```python
from build123d import *

# Parameters (mm, degrees)
SKETCH_1_R          = 5
EXTRUDE_1_DEPTH     = 5
SKETCH_3_W          = 5
SKETCH_3_H          = 8
EXTRUDE_2_DEPTH     = 15
SKETCH_2_R          = 2
CUT_EXTRUDE_1_DEPTH = 30
SKETCH_6_W          = 5
SKETCH_6_H          = 8
EXTRUDE_4_DEPTH     = 25
SKETCH_7_W          = 5
SKETCH_7_H          = 8
EXTRUDE_5_DEPTH     = 21
SKETCH_8_W          = 15
SKETCH_8_H          = 15
EXTRUDE_6_DEPTH     = 5
FILLET_2_R          = 2
SKETCH_9_R          = 2.15
CUT_EXTRUDE_2_DEPTH = 10
FILLET_3_R          = 5


with BuildPart() as part:
    # 草图1 → 凸台-拉伸1 (new body)
    with BuildSketch(Plane.XY):
        Circle(SKETCH_1_R)
    extrude(amount=EXTRUDE_1_DEPTH)

    # 草图3 → 凸台-拉伸2 (add)
    with BuildSketch(Plane(origin=(0, 0, 0), x_dir=(0, 0, -1), z_dir=(1, 0, 0))):
        with Locations((-2.5, 0)):
            Rectangle(SKETCH_3_W, SKETCH_3_H)
    extrude(amount=EXTRUDE_2_DEPTH)

    # 草图2 → 切除-拉伸1 (cut)
    with BuildSketch(Plane.XY.offset(5)):
        Circle(SKETCH_2_R)
    extrude(amount=-CUT_EXTRUDE_1_DEPTH, mode=Mode.SUBTRACT)

    # 草图6 → 凸台-拉伸4 (add)
    with BuildSketch(Plane.XY.offset(5)):
        with Locations((12.5, 0)):
            Rectangle(SKETCH_6_W, SKETCH_6_H)
    extrude(amount=EXTRUDE_4_DEPTH)

    # 草图7 → 凸台-拉伸5 (add)
    with BuildSketch(Plane(origin=(15, 0, 0), x_dir=(0, 0, -1), z_dir=(1, 0, 0))):
        with Locations((-27.5, 0)):
            Rectangle(SKETCH_7_W, SKETCH_7_H)
    extrude(amount=EXTRUDE_5_DEPTH)

    # 镜向2: part across plane


with BuildPart() as part_1:
    add(part.part)
    add(part.part.mirror(Plane(origin=(36, 0, 0), x_dir=(0, 0, 1), z_dir=(1, 0, 0))))

    # 草图8 → 凸台-拉伸6 (add)
    with BuildSketch(Plane.XY.offset(30)):
        with Locations((36, 0)):
            Rectangle(SKETCH_8_W, SKETCH_8_H)
    extrude(amount=-EXTRUDE_6_DEPTH)

    # 圆角2
    fillet_2_edges = [part_1.edges().sort_by_distance(p)[0] for p in [
        (28.5, -7.5, 27.5),
        (43.5, 7.5, 27.5),
        (28.5, 7.5, 27.5),
        (43.5, -7.5, 27.5),
    ]]
    fillet(fillet_2_edges, radius=FILLET_2_R)

    # 草图9 → 切除-拉伸2 (cut)
    with BuildSketch(Plane.XY.offset(30)):
        with Locations((36, 0)):
            Circle(SKETCH_9_R)
    extrude(amount=-CUT_EXTRUDE_2_DEPTH, mode=Mode.SUBTRACT)

    # 圆角3
    fillet_3_edges = [part_1.edges().sort_by_distance(p)[0] for p in [
        (10, 0, 5),
        (10, 0, 30),
        (15, 0, 25),
        (57, 0, 25),
        (62, 0, 5),
        (62, 0, 30),
    ]]
    fillet(fillet_3_edges, radius=FILLET_3_R)


solid = part_1.part
```
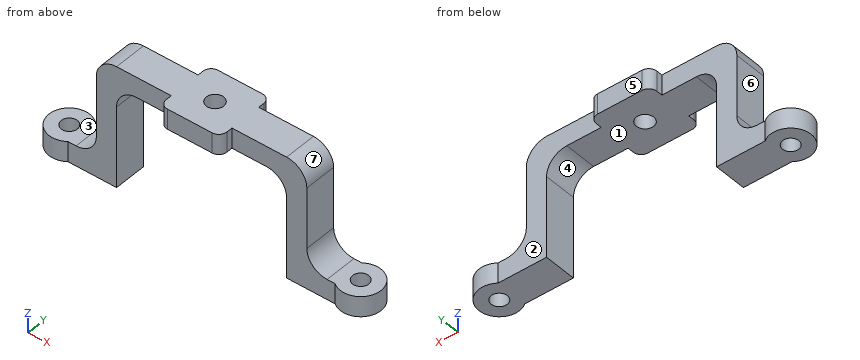
For this review, take the finished solid that the model builds, in its own axes (mm). Face numbers are marked on the shaded views. A direction names the side the tool comes from. Give positions to 0.01 mm unless a question says otherwise; leave off trailing zeros. Write each loop counter-clockwise with the first axis right and the second up, starting at its lowest first coordinate (ties: lowest second). Pieces come first, ordered by that corner, then holes.
Item 1: The part is to be moulded in two halves that separate along X. For the marked faces 4, 5, 6 and 7, say which applies: +X half, -X half, draft (parallel to the pull), parting line (faces both ways), or undercut.
Item 2: Take a section at C-C (z = 27.25). Give the boundary of the cut face in (x, y), and give its area (3 significant figures).
Item 3: Take a section at D-D (x = 55.5). Give the boundary of the cut face in (y, z), and give its area (3 significant figures).
Item 4: Take a section at A-A (z = 17.25). Give the boundary of the cut face in (x, y).
Item 5: Wall thickness on probe 1 along X at (y, z) = (2.75, 12); probe 2 along Z at (x, y) = (31.5, 6.25); probe 3 along Y at (x, z) = (12.5, 17.75): over which ranges is each line inside the solid? List them lowest first.
Item 6: Machinability: for the marked faces 1, 2 and 3, which of the approach directions +Z, -Z, +X, -X, +Y, -Y give a long, thin tool a straight path to every point of the face, cutting with its end or side? Answer none if there is none.
Item 7: Take a section at B-B (x = 72). Give the boundary of the cut face in (y, z), and give its area (3 significant figures).
Item 8: Insertion check: P1, Ø1.2, axis at y = 4.5, z = 27, coming from the +X side; P2, Ø6, axis at x = 11, z = 22, coming from the -Y side; P3, Ø6.5, axis at y = 1.5, z = 14.5, coming from the +X side; P4, Ø3.5, axis at x = 0, y = 0, coming from the -Z side. Each pin has a flat end and moves straight along its axis. Give the tip position at first contact, or say it passes through.
Established:
1. face 4: undercut
1. face 5: draft
1. face 6: -X half
1. face 7: +X half
2. outline: (10.53, -4) - (28.5, -4) - (28.5, -5.5) arc R2 ccw to (30.5, -7.5) - (41.5, -7.5) arc R2 ccw to (43.5, -5.5) - (43.5, -4) - (61.47, -4) - (61.47, 4) - (43.5, 4) - (43.5, 5.5) arc R2 ccw to (41.5, 7.5) - (30.5, 7.5) arc R2 ccw to (28.5, 5.5) - (28.5, 4) - (10.53, 4) - close; hole circle Ø4.3 at (36, 0)
2. area: 494 mm2
3. outline: (-4, 23.57) - (4, 23.57) - (4, 30) - (-4, 30) - close
3. area: 51.4 mm2
4. outline: (10, -4) - (15, -4) - (15, 4) - (10, 4) - close; (57, -4) - (62, -4) - (62, 4) - (57, 4) - close
5. probe 1: x = 10 to 15, 57 to 62
5. probe 2: z = 25 to 30
5. probe 3: y = -4 to 4
6. face 1: -Z, +Y, -Y
6. face 2: +Z, -Z, +Y
6. face 3: +Z, -X, +Y, -Y
7. outline: (-5, 0) - (-2, 0) - (-2, 5) - (-5, 5) - close; (2, 0) - (5, 0) - (5, 5) - (2, 5) - close
7. area: 30.0 mm2
8. P1: stops at x = 61.71
8. P2: stops at y = -4
8. P3: stops at x = 62
8. P4: passes through
